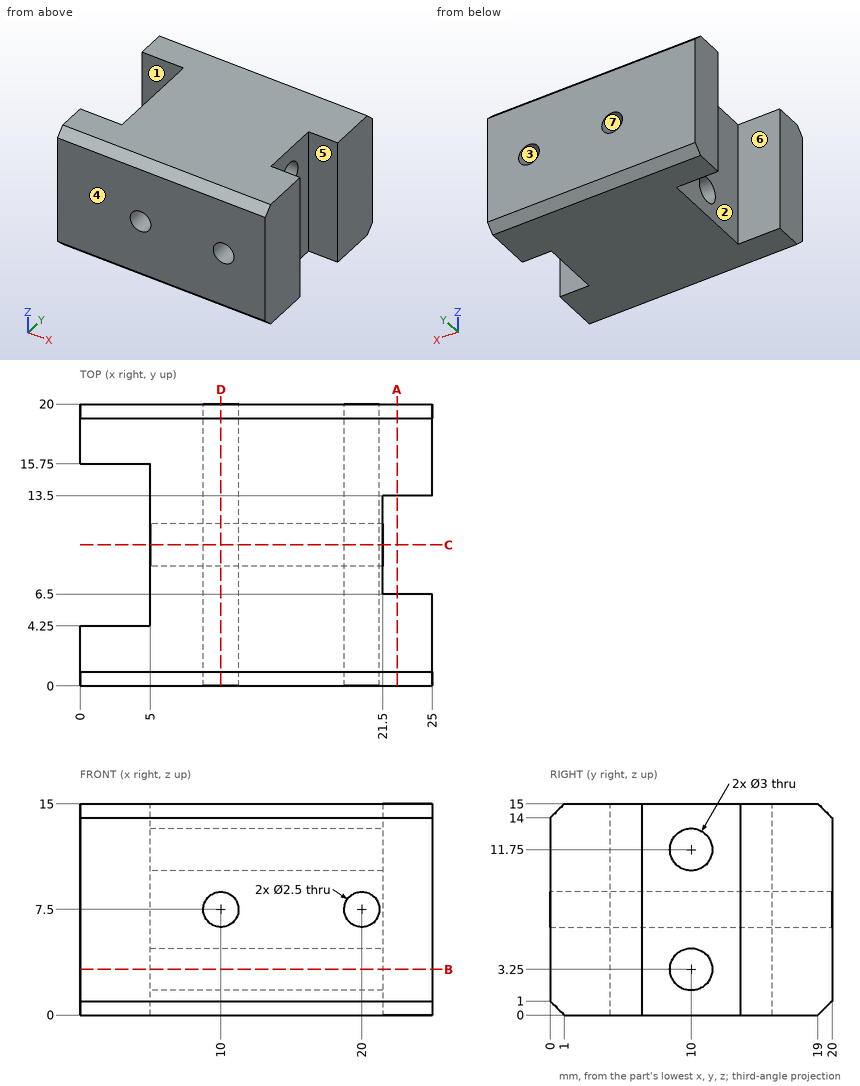
Drawing for the job (mm, zero at the part's lowest x, y, z). A direction names the side the tool comes from. Give positions to 0.01 mm unless a question says otherwise; leave off trailing zeros. Loops run counter-clockwise (first coordinate to the right, second up) from the corner with the lowest first, then second, coordinate; pieces in that order, holes last. Notation, with made-up numbers: (-11.5, 47.25) - (15.5, 47.25) arc R11 ccw to (15.5, 58.25) - close; hole circle Ø2 at (53.25, 5.25). An arc over 180 degrees is marked (long way). Write item = value, one per line. Start each with the question number.
1) Drop flat-ended pins along their axis: pin 1 Ø6 at (y, z) = (12, 9.5) entering from -X; pin 2 Ø5 at (y, z) = (10, 3.25) entering from +X. Give the stop position or say it passes through.
2) Band-saw the part on D-D on x = 10. Give the cut face in (y, z).
3) Band-saw the part on B-B on z = 3.25. Give the cut face in (x, y).
4) Pull direction Y, two halves, no side cores. Call the marked faces 1, 2, 3 and 4: +Y half, -Y half, draft (parallel to the pull), parting line (faces both ways), or undercut.
5) Band-saw the part on A-A on x = 22.5. Give the cut face in (y, z), plus the area to 3 significant figures.
6) Band-saw the part on C-C on y = 10. Give the cut face in (x, z).
7) Probe probe 1 along X at (y, z) = (6, 7.5); probe 2 along Y at (x, z) = (23.75, 9.25); probe 3 along X at (y, z) = (16, 7.25). List the from-to ranges inside material, lowest first. Write a range as from..to.
8) Tool access for the marked faces 5, 6 and 7: list every direction of +Z, -Z, +X, -X, +Y, -Y with a clear straight run to the whole face (end or side of a thin tool).
Final values:
q1.pin_1 = 5
q1.pin_2 = 21.5
q2.outline = (0, 1) - (1, 0) - (19, 0) - (20, 1) - (20, 6.25) - (0, 6.25) - close; (0, 8.75) - (20, 8.75) - (20, 14) - (19, 15) - (1, 15) - (0, 14) - close; hole circle Ø3 at (10, 3.25); hole circle Ø3 at (10, 11.75)
q3.outline = (0, 0) - (25, 0) - (25, 6.5) - (21.5, 6.5) - (21.5, 8.5) - (5, 8.5) - (5, 4.25) - (0, 4.25) - close; (0, 15.75) - (5, 15.75) - (5, 11.5) - (21.5, 11.5) - (21.5, 13.5) - (25, 13.5) - (25, 20) - (0, 20) - close
q4.face_1 = undercut
q4.face_2 = undercut
q4.face_3 = draft
q4.face_4 = -Y half
q5.outline = (0, 1) - (1, 0) - (6.5, 0) - (6.5, 15) - (1, 15) - (0, 14) - close; (13.5, 0) - (19, 0) - (20, 1) - (20, 14) - (19, 15) - (13.5, 15) - close
q5.area = 193 mm²
q6.outline = (5, 0) - (21.5, 0) - (21.5, 1.75) - (5, 1.75) - close; (5, 4.75) - (21.5, 4.75) - (21.5, 10.25) - (5, 10.25) - close; (5, 13.25) - (21.5, 13.25) - (21.5, 15) - (5, 15) - close; hole circle Ø2.5 at (10, 7.5); hole circle Ø2.5 at (20, 7.5)
q7.probe_1 = 5..8.75, 11.25..18.75, 21.25..25
q7.probe_2 = 0..6.5, 13.5..20
q7.probe_3 = 0..8.78, 11.22..18.78, 21.22..25
q8.face_5 = +Z, -Z, +X
q8.face_6 = +Z, -Z, -X
q8.face_7 = +Y, -Y
